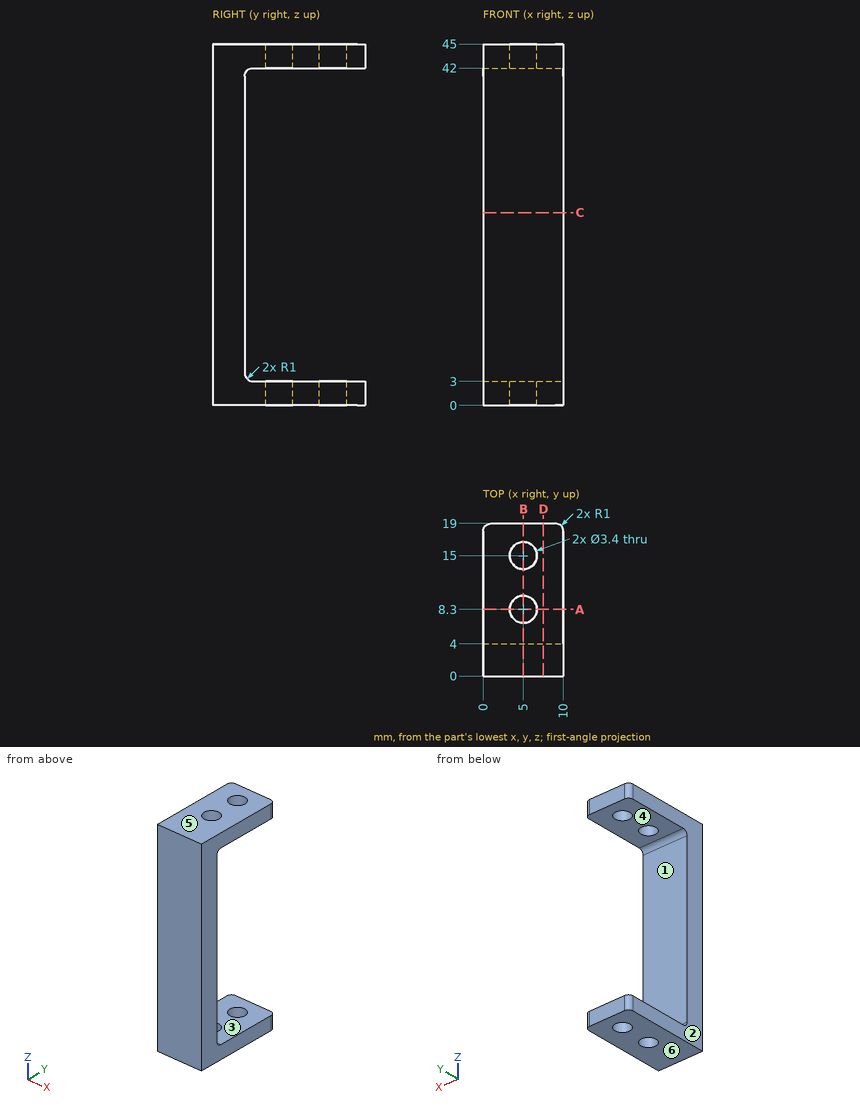
For this review, use the dimensioned drawing (mm, ordinates from the lowest corner) and the shaded views. A direction names the side the tool comes from. Give positions to 0.01 mm unless a question says otherwise; leave off trailing zeros. Loops run counter-clockwise (first coordinate to the right, second up) from the corner with the lowest first, then second, coordinate; pieces in that order, holes last. Notation, with made-up numbers: (-6.5, -32.5) -> (40.5, -32.5) arc R14 cw to (40.5, -7.5) -> close; hole circle Ø7 at (35.5, 51). An arc over 180 degrees is marked (long way). One line per question, with ' | ' between items. Start each with the question number.
(1) Draft analysis for pull direction Z (two halves, no side actions). For the marked faces 3, 4, 5 and 6, state which applies: +Z half, -Z half, draft (parallel to the pull), parting line (faces both ways), or undercut.
(2) We need section A-A (y = 8.3). State the section outline as (x, z) points.
(3) We need section B-B (x = 5). State the section outline as (y, z) points, and give its area (3 significant figures).
(4) We need section D-D (x = 7.5). State the section outline as (y, z) points.
(5) Insertion check: P1, Ø1, axis at x = 2, z = 8.5, coming from the +Y side; P2, Ø1, axis at x = 8.5, z = 12.5, coming from the -Y side. Each pin has a flat end and moves straight along its axis. Give the tip position at first contact, or say it passes through.
(6) For the marked faces 1 and 2, list the 3-axis set-ups (+Z, -Z, +X, -X, +Y, -Y) from which the entire face can be reached by the end or side of a thin tool; tool diameter is ignored.
(7) We need section C-C (z = 24). State the section outline as (x, y) points, and give its area (3 significant figures).
(8) For line 1 (Y direction, x = 5, z = 44.3); line 2 (X direction, y = 15, z = 43.6); line 3 (Z direction, x = 7.75, y = 9.25), list the stretches that pass through material, from the lowest coordinate up.
The answers:
1) face 3: undercut | face 4: undercut | face 5: +Z half | face 6: -Z half
2) outline: (0, 0) -> (3.3, 0) -> (3.3, 3) -> (0, 3) -> close; (0, 42) -> (3.3, 42) -> (3.3, 45) -> (0, 45) -> close; (6.7, 0) -> (10, 0) -> (10, 3) -> (6.7, 3) -> close; (6.7, 42) -> (10, 42) -> (10, 45) -> (6.7, 45) -> close
3) outline: (0, 0) -> (6.6, 0) -> (6.6, 3) -> (5, 3) arc R1 cw to (4, 4) -> (4, 41) arc R1 cw to (5, 42) -> (6.6, 42) -> (6.6, 45) -> (0, 45) -> close; (10, 0) -> (13.3, 0) -> (13.3, 3) -> (10, 3) -> close; (10, 42) -> (13.3, 42) -> (13.3, 45) -> (10, 45) -> close; (16.7, 0) -> (19, 0) -> (19, 3) -> (16.7, 3) -> close; (16.7, 42) -> (19, 42) -> (19, 45) -> (16.7, 45) -> close | area: 230 mm^2
4) outline: (0, 0) -> (19, 0) -> (19, 3) -> (5, 3) arc R1 cw to (4, 4) -> (4, 41) arc R1 cw to (5, 42) -> (19, 42) -> (19, 45) -> (0, 45) -> close
5) P1: stops at y = 4 | P2: stops at y = 0
6) face 1: +X, -X, +Y | face 2: +Z, -Z, -X, +Y, -Y
7) outline: (0, 0) -> (10, 0) -> (10, 4) -> (0, 4) -> close | area: 40.0 mm^2
8) line 1: y = 0 to 6.6, 10 to 13.3, 16.7 to 19 | line 2: x = 0 to 3.3, 6.7 to 10 | line 3: z = 0 to 3, 42 to 45
